Geometry: final body of the model. Coordinates: model frame, mm. A direction names the side the tool comes from. Coordinates: 2 decimals unless noted, no trailing zeros. Order: outer loops, then holes, each group sorted by start corner. A loop starts at its lowest first (then second) coordinate and runs counter-clockwise, first axis right, second up. Notation, with made-up numbers: M 15,37.25 L 45,37.25 A21 cw 45,41.25 Z; hole C -9.75,39 d10. An arc over 180 degrees is marked long. Use CSV: the item, a comma, the result in double quotes. Start each with the question number.
1. First-contact query: P1, Ø5, axis at x = 4, z = -2, coming from the +Y side; P2, Ø3, axis at y = 7, z = -2, coming from the +X side; P3, Ø1.8, axis at x = 0, z = 0, coming from the -Y side. Flat tips, straight axial feed; report the tip coordinate or a pass-through.
2. Section query D-D on y = 9. Return the cut outline in (x, z), and give its area (3 significant figures).
3. Set-up query: faces 1 (the flat face through (16.5, 5, 0)), 2 (the flat face through (8, 0, 0)). Return all of +Z, -Z, +X, -X, +Y, -Y with unobstructed straight access to the full face (end or side cutting, diameter ignored); none if empty.
4. Section query B-B on y = 3. Return the cut outline in (x, z).
5. Section query A-A on z = 0. Return the cut outline in (x, y), and give its area (3 significant figures).
6. Pull-direction query (Z, two-part tool) for faces 3 (the flat face through (12.8, 10, -0.1)), 4 (the cylindrical face through (-5, 3, 0)), 5 (the cylindrical face through (13, 5, 0)); classes: pulls with the +Z half, pulls with the -Z half, needs draft (parallel to the pull), parting line crosses it, or undercut.
7. Material intervals for line 1 (X direction, y = 1.55, z = 0); line 2 (X direction, y = 7.75, z = 0); line 3 (Z direction, x = 15, y = 4), sorted ascending.
8. Section query C-C on x = 0.5. Return the cut outline in (y, z), and give its area (3 significant figures).
from build123d import *
from build123d.topology import SkipClean

# Parameters (mm, degrees)
SKETCH1_R           = 1
BOSS_EXTRUDE1_DEPTH = 6
SKETCH2_R           = 5
BOSS_EXTRUDE2_DEPTH = 4
CUT_EXTRUDE1_DEPTH  = 23.912878475


with BuildPart() as part:
    # Sketch1 → Boss-Extrude1 (new body)
    with BuildSketch(Plane(origin=(0, 0, 0), x_dir=(1, 0, 0), z_dir=(0, 1, 0))):
        with BuildLine():
            Line((0, 5), (15, 5))
            ThreePointArc((15, 5), (20, 0), (15, -5))
            Line((15, -5), (0, -5))
            ThreePointArc((0, -5), (-5, 0), (0, 5))
        make_face()
        with Locations(Location((0, 0, 0), (0, 0, 270))):
            Circle(SKETCH1_R, mode=Mode.SUBTRACT)
    extrude(amount=BOSS_EXTRUDE1_DEPTH)

    # Sketch2 → Boss-Extrude2 (add)
    with SkipClean():  # the faces are left unmerged after this step: merging them gives an invalid solid
        with BuildSketch(Plane(origin=(0, 6, 0), x_dir=(1, 0, 0), z_dir=(0, 1, 0))):
            with Locations(Location((15, 0, 0), (0, 0, 270))):
                Circle(SKETCH2_R)
        extrude(amount=BOSS_EXTRUDE2_DEPTH)
    add(part.part.scale(1), mode=Mode.REPLACE)  # the faces are merged on a copy

    # Sketch3 → Cut-Extrude1 (cut, through all)
    with BuildSketch(Plane(origin=(0, 10, 0), x_dir=(1, 0, 0), z_dir=(0, 1, 0))):
        with BuildLine():
            Line((16.5, -1.322875656), (16.5, 1.322875656))
            ThreePointArc((16.5, 1.322875656), (13, 0), (16.5, -1.322875656))
        make_face()
    extrude(amount=-CUT_EXTRUDE1_DEPTH, mode=Mode.SUBTRACT)


solid = part.part
Results list:
1,P1,"stops at y = 6"
1,P2,"stops at x = 19.97"
1,P3,"passes through"
2,outline,"C 15,0 d10; hole M 16.5,-1.32 L 16.5,1.32 A2 ccw long Z"
2,area,"66.9 mm²"
3,face 1,"+Y, -Y"
3,face 2,"+Z, -Z, +X, -X, -Y"
4,outline,"M 0,-5 L 15,-5 A5 ccw 15,5 L 0,5 A5 ccw Z; hole C 0,0 d2; hole M 16.5,-1.32 L 16.5,1.32 A2 ccw long Z"
5,outline,"M -5,0 L -1,0 L -1,6 L -5,6 Z; M 1,0 L 13,0 L 13,10 L 10,10 L 10,6 L 1,6 Z; M 16.5,0 L 20,0 L 20,10 L 16.5,10 Z"
5,area,"143 mm²"
6,face 3,"needs draft"
6,face 4,"parting line crosses it"
6,face 5,"undercut"
7,line 1,"x = -5 to -1, 1 to 13, 16.5 to 20"
7,line 2,"x = 10 to 13, 16.5 to 20"
7,line 3,"z = -5 to -2, 2 to 5"
8,outline,"M 0,-5 L 6,-5 L 6,-0.87 L 0,-0.87 Z; M 0,0.87 L 6,0.87 L 6,5 L 0,5 Z"
8,area,"49.6 mm²"
